Read the model definition and answer for the solid it produces. Units are mm, in the model's axes. A direction names the side the tool comes from. Round coordinates to 2 decimals unless told otherwise and drop trailing zeros. Order: outer loops, then holes, each group sorted by start corner. A loop starts at its lowest first (then second) coordinate and runs counter-clockwise, first axis right, second up.
from build123d import *

# Parameters (mm, degrees)
EXTRUDE_2_DEPTH     = 42
SKETCH_2_R          = 1.35
CUT_EXTRUDE_1_DEPTH = 45
CUT_EXTRUDE_2_DEPTH = 45
SKETCH_4_W          = 4
SKETCH_4_H          = 46.1
EXTRUDE_3_DEPTH     = 4
SKETCH_5_W          = 2
SKETCH_5_H          = 46.1
EXTRUDE_4_DEPTH     = 42
SKETCH_6_R          = 1.25
CUT_EXTRUDE_3_DEPTH = 10


with BuildPart() as part:
    # Sketch 1 → Extrude 2 (new body)
    with BuildSketch(Plane.XY):
        with BuildLine():
            Line((-14.5, -41.5), (-14.5, 11.5))
            Line((-14.5, 11.5), (-14.5, 13))
            Line((-14.5, 13), (-15, 13))
            Line((-15, 13), (-20.1, 5.5))
            Line((-20.1, 5.5), (-20.1, -40.6))
            Line((-20.1, -40.6), (-15, -48.1))
            Line((-15, -48.1), (15, -48.1))
            Line((15, -48.1), (20.1, -40.6))
            Line((20.1, -40.6), (20.1, 5.5))
            Line((20.1, 5.5), (15, 13))
            Line((15, 13), (14.5, 13))
            Line((14.5, 13), (14.5, 11.5))
            Line((14.5, 11.5), (14.5, -41.5))
            ThreePointArc((14.5, -41.5), (14.207106781, -42.207106781), (13.5, -42.5))
            Line((13.5, -42.5), (-13.5, -42.5))
            ThreePointArc((-13.5, -42.5), (-14.207106781, -42.207106781), (-14.5, -41.5))
        make_face()
    extrude(amount=EXTRUDE_2_DEPTH)

    # Sketch 2 → Cut-Extrude 1 (cut)
    with BuildSketch(Plane(origin=(0, 0, 0), x_dir=(-1, 0, 0), z_dir=(0, 0, -1))):
        with Locations((-11, -45.405560676)):
            Circle(SKETCH_2_R)
        with Locations((11, -45.405560676)):
            Circle(SKETCH_2_R)
        with Locations((17.3, 3.87)):
            Circle(SKETCH_2_R)
        with Locations((17.3, -18.13)):
            Circle(SKETCH_2_R)
        with Locations((-17.3, 3.87)):
            Circle(SKETCH_2_R)
        with Locations((-17.3, -18.13)):
            Circle(SKETCH_2_R)
    extrude(amount=-CUT_EXTRUDE_1_DEPTH, mode=Mode.SUBTRACT)

    # Sketch 3 → Cut-Extrude 2 (cut)
    with BuildSketch(Plane(origin=(20.1, 0, 0), x_dir=(0, 0, -1), z_dir=(1, 0, 0))):
        Polygon((-38, 5.5), (-38, -40.6), (-38, -48.1), (-4, -48.1), (-4, -40.6), (-4, 5.5), (-4, 13), (-38, 13), align=None)
    extrude(amount=-CUT_EXTRUDE_2_DEPTH, mode=Mode.SUBTRACT)


with BuildPart() as cut_extrude_2_piece_1:
    # of the separate pieces the step leaves, piece 1, a body of its own (cut_extrude_2_pieces)
    add(part.part.solids().sort_by_distance((-14.5, -41.5, 38))[0])



with BuildPart() as cut_extrude_2_piece_2:
    # of the separate pieces the step leaves, piece 2, a body of its own (cut_extrude_2_pieces)
    add(part.part.solids().sort_by_distance((-14.5, -41.5, 0))[0])


with BuildPart() as cut_extrude_2_piece_1_1:
    add(cut_extrude_2_piece_1.part)

    add(cut_extrude_2_piece_2.part)  # Extrude 3 merges Cut-Extrude 2 piece 2
    # Sketch 4 → Extrude 3 (add)
    with BuildSketch(Plane(origin=(20.1, 0, 0), x_dir=(0, 0, -1), z_dir=(1, 0, 0))):
        with Locations((-40, -17.55)):
            Rectangle(SKETCH_4_W, SKETCH_4_H)
        with Locations((-2, -17.55)):
            Rectangle(SKETCH_4_W, SKETCH_4_H)
    extrude(amount=EXTRUDE_3_DEPTH)

    # Sketch 5 → Extrude 4 (add)
    with BuildSketch(Plane.XY.offset(42)):
        with Locations((25.1, -17.55)):
            Rectangle(SKETCH_5_W, SKETCH_5_H)
    extrude(amount=-EXTRUDE_4_DEPTH)

    # Sketch 6 → Cut-Extrude 3 (cut)
    with BuildSketch(Plane(origin=(26.1, 0, 0), x_dir=(0, 0, -1), z_dir=(1, 0, 0))):
        with Locations((-21, -17.55)):
            Circle(SKETCH_6_R)
        with Locations((-11, -17.55)):
            Circle(SKETCH_6_R)
        with Locations((-31, -17.55)):
            Circle(SKETCH_6_R)
        with Locations((-31, -7.55)):
            Circle(SKETCH_6_R)
        with Locations((-21, -7.55)):
            Circle(SKETCH_6_R)
        with Locations((-11, -7.55)):
            Circle(SKETCH_6_R)
        with Locations((-31, -27.55)):
            Circle(SKETCH_6_R)
        with Locations((-21, -27.55)):
            Circle(SKETCH_6_R)
        with Locations((-11, -27.55)):
            Circle(SKETCH_6_R)
    extrude(amount=-CUT_EXTRUDE_3_DEPTH, mode=Mode.SUBTRACT)


solid = cut_extrude_2_piece_1_1.part
Q1. For a pull along Y with two mould halves and no side action, classify faces 4 (the face through (-15.95, 3.93, 1.97)), 5 (the face through (-17.586, -44.298, 39.972)), 6 (the face through (26.1, -18, 26)) as released by +Y, released by -Y, zero draft, split by the parting line, or undercut.
Outcome:
face 4: undercut
face 5: released by -Y
face 6: zero draft
Q2. A cutting plane is placed at B-B, the plane y = -7.55. Give the vertices of the cut face in (x, z).
Outcome:
outline: (-20.1, 0) - (-14.5, 0) - (-14.5, 4) - (-20.1, 4) - close; (-20.1, 38) - (-14.5, 38) - (-14.5, 42) - (-20.1, 42) - close; (14.5, 0) - (26.1, 0) - (26.1, 9.75) - (24.1, 9.75) - (24.1, 4) - (14.5, 4) - close; (14.5, 38) - (24.1, 38) - (24.1, 32.25) - (26.1, 32.25) - (26.1, 42) - (14.5, 42) - close; (24.1, 12.25) - (26.1, 12.25) - (26.1, 19.75) - (24.1, 19.75) - close; (24.1, 22.25) - (26.1, 22.25) - (26.1, 29.75) - (24.1, 29.75) - close
Q3. A cutting plane is placed at A-A, the plane y = -31.5. Give the vertices of the cut face in (x, z), plus the area to 3 significant figures.
Outcome:
outline: (-20.1, 0) - (-14.5, 0) - (-14.5, 4) - (-20.1, 4) - close; (-20.1, 38) - (-14.5, 38) - (-14.5, 42) - (-20.1, 42) - close; (14.5, 0) - (26.1, 0) - (26.1, 42) - (14.5, 42) - (14.5, 38) - (24.1, 38) - (24.1, 4) - (14.5, 4) - close
area: 206 mm2
Q4. Flat-ended cylindrical pins translate along their axes: pin 1 (3 mm diameter, centred on y = -7.55, z = 31, fed in from -X); pin 2 (3.5 mm diameter, centred on x = -17.3, y = 3.87, fed in from +Z); pin 3 (12 mm diameter, centred on x = -4, z = 36, fed in from +Y). Find the tip coordinate at first contact, or state that the pin passes through.
Outcome:
pin 1: stops at x = 24.1
pin 2: stops at z = 42
pin 3: stops at y = -42.5
Q5. Straight lines are drawn through the part: probe 1 along Y at (x, z) = (25.6, 31); probe 2 along Z at (x, y) = (24, -17); probe 3 along Z at (x, y) = (25, -27). For each, find the intervals that lie inside material, in ascending order.
Outcome:
probe 1: y = -40.6 to -28.8, -26.3 to -18.8, -16.3 to -8.8, -6.3 to 5.5
probe 2: z = 0 to 4, 38 to 42
probe 3: z = 0 to 9.88, 12.12 to 19.88, 22.12 to 29.88, 32.12 to 42
Q6. For faces 1 (the face through (-14.5, -15, 40)), 2 (the face through (25.114, -16.705, 11.921)), 3 (the face through (24.4, -40.6, 21.3)), determine the directions among +Z, -Z, +X, -X, +Y, -Y from which every point of the face is accessible in a straight line to the end or side of a thin tool.
Outcome:
face 1: +Z, -Z, +Y
face 2: +X, -X
face 3: +Z, -Z, +X, -Y
Q7. A cutting plane is placed at D-D, the plane x = 11. Give the vertices of the cut face in (y, z), plus the area to 3 significant figures.
Outcome:
outline: (-48.1, 0) - (-46.76, 0) - (-46.76, 4) - (-48.1, 4) - close; (-48.1, 38) - (-46.76, 38) - (-46.76, 42) - (-48.1, 42) - close; (-44.06, 0) - (-42.5, 0) - (-42.5, 4) - (-44.06, 4) - close; (-44.06, 38) - (-42.5, 38) - (-42.5, 42) - (-44.06, 42) - close
area: 23.2 mm2
Q8. A cutting plane is placed at C-C, the plane z = 21. Give the vertices of the cut face in (x, y), plus the area to 3 significant figures.
Outcome:
outline: (24.1, -40.6) - (26.1, -40.6) - (26.1, -28.8) - (24.1, -28.8) - close; (24.1, -26.3) - (26.1, -26.3) - (26.1, -18.8) - (24.1, -18.8) - close; (24.1, -16.3) - (26.1, -16.3) - (26.1, -8.8) - (24.1, -8.8) - close; (24.1, -6.3) - (26.1, -6.3) - (26.1, 5.5) - (24.1, 5.5) - close
area: 77.2 mm2
